from build123d import *

# Parameters (mm, degrees)
BOSS_EXTRUDE1_DEPTH                               = 3
CSK_FOR_M2_5_FLAT_HEAD_MACHINE_SCREW1_D           = 2.9
CSK_FOR_M2_5_FLAT_HEAD_MACHINE_SCREW1_CSINK_D     = 5.5
CSK_FOR_M2_5_FLAT_HEAD_MACHINE_SCREW1_CSINK_ANGLE = 90
FILLET1_R                                         = 3.75


with BuildPart() as part:
    # Sketch1 → Boss-Extrude1 (new body)
    with BuildSketch(Plane(origin=(0, 0, 0), x_dir=(1, 0, 0), z_dir=(0, 1, 0))):
        with BuildLine():
            Line((0, 0), (0, -20))
            ThreePointArc((0, -20), (31.599050619, -18.748037795), (63, -15))
            Line((63, -15), (70, -3))
            Line((70, -3), (30, 5))
            Line((30, 5), (20, 0))
            Line((20, 0), (0, 0))
        make_face()
    boss_extrude1 = extrude(amount=BOSS_EXTRUDE1_DEPTH)

    # CSK for M2.5 Flat Head Machine Screw1 (through all)
    with Locations(Plane(origin=(0, 3, 0), x_dir=(1, 0, 0), z_dir=(0, 1, 0))):
        with Locations((29, 0), (30, -12.5)):
            csk_for_m2_5_flat_head_machine_screw1 = CounterSinkHole(CSK_FOR_M2_5_FLAT_HEAD_MACHINE_SCREW1_D / 2, CSK_FOR_M2_5_FLAT_HEAD_MACHINE_SCREW1_CSINK_D / 2, counter_sink_angle=CSK_FOR_M2_5_FLAT_HEAD_MACHINE_SCREW1_CSINK_ANGLE)

    # Mirror1: Boss-Extrude1, CSK for M2.5 Flat Head Machine Screw1 across plane
    add(boss_extrude1.mirror(Plane(origin=(0, 0, 0), x_dir=(0, 0, 1), z_dir=(1, 0, 0))))
    add(csk_for_m2_5_flat_head_machine_screw1.mirror(Plane(origin=(0, 0, 0), x_dir=(0, 0, 1), z_dir=(1, 0, 0))), mode=Mode.SUBTRACT)

    # Fillet1
    fillet1_edges = [part.edges().sort_by_distance(p)[0] for p in [
        (20, 1.5, 0),
        (30, 1.5, -5),
        (70, 1.5, 3),
        (63, 1.5, 15),
        (-20, 1.5, 0),
        (-30, 1.5, -5),
        (-70, 1.5, 3),
        (-63, 1.5, 15),
    ]]
    fillet(fillet1_edges, radius=FILLET1_R)


solid = part.part
Design review of the part built by this model. Coordinates are the model's own, in mm. A direction names the side the tool comes from. Coordinates: 2 decimals unless noted, no trailing zeros. Loops run counter-clockwise (first coordinate to the right, second up) from the corner with the lowest first, then second, coordinate; pieces in that order, holes last. Notation, with made-up numbers: M 23.5,48.25 L 69.5,48.25 A15 cw 69.5,59.25 Z; hole C 60.25,-2.75 d2. An arc over 180 degrees is marked long. Use one line per item in the form item = value.
(1) Draft analysis for pull direction X (two halves, no side actions). For faces 3 (the face through (-24.88, 1.48, -2.44)), 4 (the face through (48.29, 1.48, -1.34)), 5 (the face through (-65.6, 1.48, 10.54)), 6 (the face through (1, 0, 7)), state which applies: pulls with the +X half, pulls with the -X half, needs draft (parallel to the pull), parting line crosses it, or undercut.
Return value:
face_3 = undercut
face_4 = pulls with the +X half
face_5 = pulls with the -X half
face_6 = needs draft
(2) For faces 1 (the face through (24.88, 1.48, -2.44)), 2 (the face through (-48.29, 1.48, -1.34)), list the 3-axis set-ups (+Z, -Z, +X, -X, +Y, -Y) from which the entire face can be reached by the end or side of a thin tool; tool diameter is ignored.
Return value:
face_1 = -Z, +Y, -Y
face_2 = -Z, -X, +Y, -Y
(3) Clearance check with a flat-ended pin moving along its axis: P1, Ø2.5, axis at x = 30, z = 12.5, coming from the -Y side. State where the tip first meets the part, or that it passes through.
Return value:
P1 = through
(4) For line 1 along Z through (x, y) = (-30, 0.75); line 2 along Z through (x, y) = (29, 0.65); line 3 along Z through (x, y) = (-4, 2.65), list the stretches that pass through material, from the lowest coordinate up. Write a range as from..to.
Return value:
line_1 = -4.78..-1.05, 1.05..11.05, 13.95..18.87
line_2 = -4.5..-1.45, 1.45..11.45, 13.55..18.95
line_3 = 0..19.98
(5) Consider section B-B (x = 39). Write out the cut boundary in (y, z), and give its area (3 significant figures).
Return value:
outline = M 0,-3.2 L 3,-3.2 L 3,18.09 L 0,18.09 Z
area = 63.9 mm2
(6) Consider section A-A (y = 0.6). Write out the cut boundary in (x, z), and give its area (3 significant figures).
Return value:
outline = M -67.35,7.54 A3.75 ccw -64.85,1.97 L -31.26,-4.75 A3.75 ccw -28.85,-4.42 L -20.79,-0.4 A3.75 cw -19.11,0 L 19.11,0 A3.75 cw 20.79,-0.4 L 28.85,-4.42 A3.75 ccw 31.26,-4.75 L 64.85,1.97 A3.75 ccw 67.35,7.54 L 63.9,13.46 A3.75 ccw 61.23,15.28 A399.4 ccw -61.23,15.28 A3.75 ccw -63.9,13.46 Z; hole C -30,12.5 d2.9; hole C -29,0 d2.9; hole C 29,0 d2.9; hole C 30,12.5 d2.9
area = 2,530 mm2
